Here's the drawing with two shaded views (mm, measured from the low corner). I have some questions. A direction names the side the tool comes from. Coordinates: 2 decimals unless noted, no trailing zeros. Write each loop counter-clockwise with the first axis right and the second up, starting at its lowest first coordinate (ties: lowest second). Pieces come first, ordered by that corner, then holes. Notation, with made-up numbers: (23.25, -23.75) -> (57.25, -23.75) arc R32 ccw to (57.25, 4.25) -> close; hole circle Ø11 at (89, 38). An arc over 180 degrees is marked (long way). Use one line per item in the form item = value.
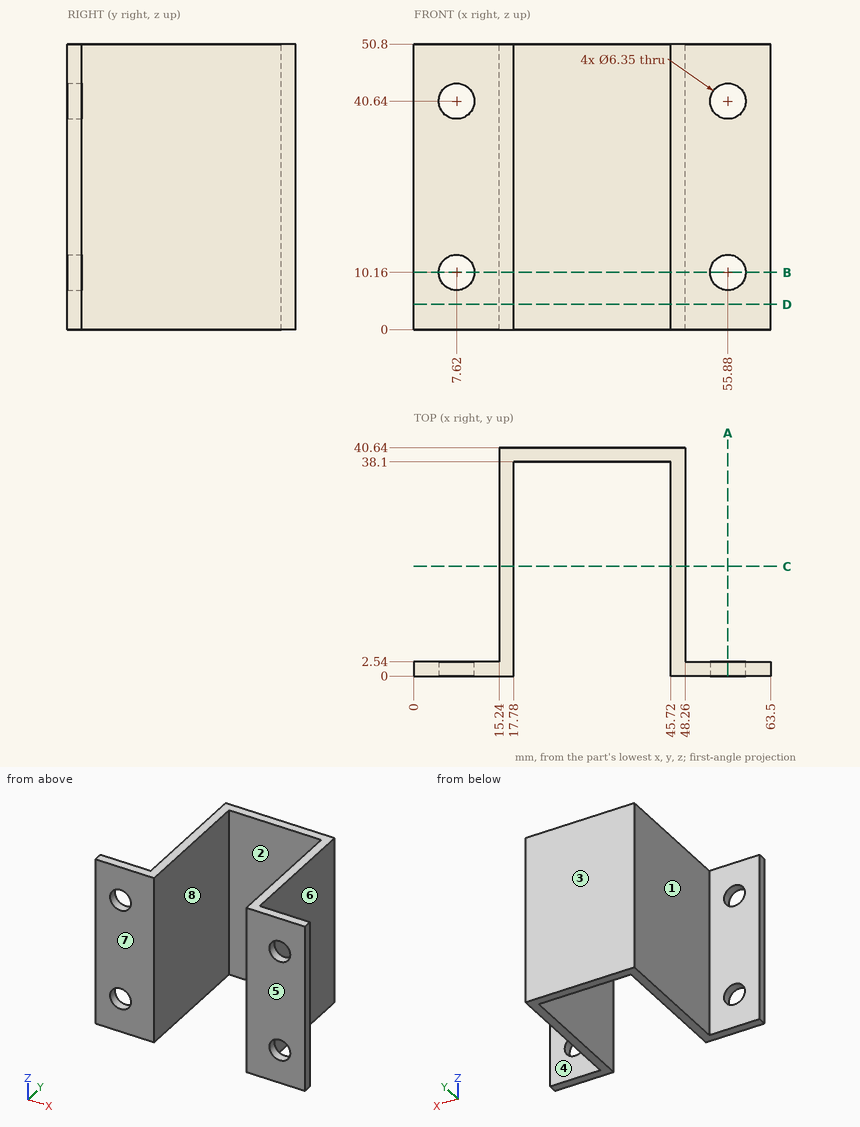
Q1. Will these pins go through, and if not, where does the flat tip stop? pin 1 (10 mm diameter, centred on y = 29, z = 38.5, fed in from -X); pin 2 (7.5 mm diameter, centred on x = 7.5, z = 24, fed in from +Y); pin 3 (12 mm diameter, centred on x = 36, z = 30, fed in from -Y).
Return value:
pin_1 = 15.24
pin_2 = 2.54
pin_3 = 38.1
Q2. Suppose I cut it at D-D (z = 4.5). Write out the boundary of the cut face in (x, y), then the cut area to 3 significant figures.
Return value:
outline = (0, 0) -> (17.78, 0) -> (17.78, 38.1) -> (45.72, 38.1) -> (45.72, 0) -> (63.5, 0) -> (63.5, 2.54) -> (48.26, 2.54) -> (48.26, 40.64) -> (15.24, 40.64) -> (15.24, 2.54) -> (0, 2.54) -> close
area = 355 mm2
Q3. Thinking about a two-plate mould opening in X: for the marked faces 6, 7 and 8, which applies, released by +X, released by -X, zero draft, split by the parting line, or undercut?
Return value:
face_6 = released by +X
face_7 = zero draft
face_8 = undercut
Q4. Suppose I cut it at A-A (x = 55.88). Write out the boundary of the cut face in (y, z) (3 decimals).
Return value:
outline = (0, 0) -> (2.54, 0) -> (2.54, 6.985) -> (0, 6.985) -> close; (0, 13.335) -> (2.54, 13.335) -> (2.54, 37.465) -> (0, 37.465) -> close; (0, 43.815) -> (2.54, 43.815) -> (2.54, 50.8) -> (0, 50.8) -> close
Q5. If I drill on line 1 (Z direction, x = 55.88, y = 1.8) (3 decimals); line 2 (X direction, y = 10, z = 4); line 3 (Z direction, x = 55, y = 1), over which ranges is the centre line in solid material (lowest first)? Write a range as from..to.
Return value:
line_1 = 0..6.985, 13.335..37.465, 43.815..50.8
line_2 = 15.24..17.78, 45.72..48.26
line_3 = 0..7.11, 13.21..37.59, 43.69..50.8
Q6. For the marked faces 1, 2, 3, 4 and 5, which set-ups out of +Z, -Z, +X, -X, +Y, -Y let a thin tool reach every point of the face, with its end or its side?
Return value:
face_1 = +Z, -Z, -X, +Y
face_2 = +Z, -Z, -Y
face_3 = +Z, -Z, +X, -X, +Y
face_4 = +Z, -Z, +X, +Y
face_5 = +Z, -Z, +X, -X, -Y
Q7. Suppose I cut it at B-B (z = 10.16). Write out the boundary of the cut face in (x, y) (3 decimals), then the cut area to 3 significant figures.
Return value:
outline = (0, 0) -> (4.445, 0) -> (4.445, 2.54) -> (0, 2.54) -> close; (10.795, 0) -> (17.78, 0) -> (17.78, 38.1) -> (45.72, 38.1) -> (45.72, 0) -> (52.705, 0) -> (52.705, 2.54) -> (48.26, 2.54) -> (48.26, 40.64) -> (15.24, 40.64) -> (15.24, 2.54) -> (10.795, 2.54) -> close; (59.055, 0) -> (63.5, 0) -> (63.5, 2.54) -> (59.055, 2.54) -> close
area = 323 mm2
Q8. Suppose I cut it at C-C (y = 19.5). Write out the boundary of the cut face in (x, z).
Return value:
outline = (15.24, 0) -> (17.78, 0) -> (17.78, 50.8) -> (15.24, 50.8) -> close; (45.72, 0) -> (48.26, 0) -> (48.26, 50.8) -> (45.72, 50.8) -> close
